Check sheet for the modelled part. Datum: model origin and axes. Units: mm. Round coordinates to 2 decimals unless told otherwise and drop trailing zeros. Write each loop counter-clockwise with the first axis right and the second up, starting at its lowest first coordinate (ties: lowest second). Pieces come first, ordered by that corner, then holes. Notation, with made-up numbers: (51.25, -21) -> (90.25, -21) arc R10 cw to (90.25, -10) -> close; hole circle Ø9 at (17, 6.25). An arc over 180 degrees is marked (long way). One line per item, written item: value. Start each with the question number.
```python
from build123d import *

# Parameters (mm, degrees)
F0_W     = 609.6
F0_H     = 609.6
F1_DEPTH = 0.79375
F2_R     = 5.55625
F3_DEPTH = 25.4
F4_R     = 7.14375
F5_DEPTH = 25.4


# Not quite as in the source:
# - a feature names something its author has since deleted; it is built from what else it names


with BuildPart() as f1:
    # F0 (on Top) → F1 (new body)
    with BuildSketch(Plane.XY):
        with Locations((304.8, 304.8)):
            Rectangle(F0_W, F0_H)
    extrude(amount=F1_DEPTH)

    # F2 (on face) → F3 (cut)
    with BuildSketch(Plane.XY.offset(0.79375)):
        with Locations((47.625, 152.4)):
            Circle(F2_R)
        with Locations((47.625, 355.6)):
            Circle(F2_R)
        with Locations((561.975, 254)):
            Circle(F2_R)
        with Locations((561.975, 457.2)):
            Circle(F2_R)
    extrude(amount=-F3_DEPTH, mode=Mode.SUBTRACT)

    # F4 (on face) → F5 (cut)
    with BuildSketch(Plane.XY.offset(0.79375)):
        with Locations((187.325, 50.8)):
            Circle(F4_R)
        with Locations((117.475, 34.925)):
            Circle(F4_R)
        with Locations((152.4, 101.6)):
            Circle(F4_R)
        with Locations((152.4, 184.15)):
            Circle(F4_R)
        with Locations((152.4, 288.925)):
            Circle(F4_R)
        with Locations((422.275, 34.925)):
            Circle(F4_R)
        with Locations((492.125, 50.8)):
            Circle(F4_R)
        with Locations((457.2, 101.6)):
            Circle(F4_R)
        with Locations((457.2, 184.15)):
            Circle(F4_R)
        with Locations((457.2, 288.925)):
            Circle(F4_R)
    extrude(amount=-F5_DEPTH, mode=Mode.SUBTRACT)


solid = f1.part
```
1. Material ranges on probe 1 along Y at (x, z) = (152.4, 0.45); probe 2 along X at (y, z) = (105, 0.3); probe 3 along Y at (x, z) = (188.5, 0.75), recorded low to high.
2. Cross-section at B-B (x = 457.2). Record the cut outline in (y, z), plus the area to 3 significant figures.
3. Cross-section at A-A (y = 50.8). Record the cut outline in (x, z), plus the area to 3 significant figures.
4. Depth check by flat-ended pin: pin 1 Ø16.5 at (x, y) = (457.2, 288.925) entering from +Z. Enter the tip coordinate at first touch or a pass-through.
5. Release check for a two-part mould opening along Y. For faces 1 (the face through (450.063, 101.914, 0.402)), 2 (the face through (301, 309, 0.794)) record: +Y half, -Y half, draft (parallel to the pull), parting line (faces both ways), or undercut.
Working result:
1. probe 1: y = 0 to 94.46, 108.74 to 177.01, 191.29 to 281.78, 296.07 to 609.6
1. probe 2: x = 0 to 146.12, 158.68 to 450.92, 463.48 to 609.6
1. probe 3: y = 0 to 43.75, 57.85 to 609.6
2. outline: (0, 0) -> (94.46, 0) -> (94.46, 0.79) -> (0, 0.79) -> close; (108.74, 0) -> (177.01, 0) -> (177.01, 0.79) -> (108.74, 0.79) -> close; (191.29, 0) -> (281.78, 0) -> (281.78, 0.79) -> (191.29, 0.79) -> close; (296.07, 0) -> (609.6, 0) -> (609.6, 0.79) -> (296.07, 0.79) -> close
2. area: 450 mm^2
3. outline: (0, 0) -> (180.18, 0) -> (180.18, 0.79) -> (0, 0.79) -> close; (194.47, 0) -> (484.98, 0) -> (484.98, 0.79) -> (194.47, 0.79) -> close; (499.27, 0) -> (609.6, 0) -> (609.6, 0.79) -> (499.27, 0.79) -> close
3. area: 461 mm^2
4. pin 1: stops at z = 0.79
5. face 1: undercut
5. face 2: draft
